Work out the finished part from the listing and answer in its coordinate system (mm). A direction names the side the tool comes from. Round coordinates to 2 decimals unless told otherwise and drop trailing zeros. Write each loop counter-clockwise with the first axis right and the second up, starting at its lowest first coordinate (ties: lowest second). Pieces come first, ordered by that corner, then holes.
from build123d import *

# Parameters (mm, degrees)
SKETCH_1_W                                = 111
SKETCH_1_H                                = 84
BOTTOM_LOWER_BASE_PLATE_3MM_DEPTH         = 3
SKETCH_3_R                                = 3
BOTTOM_LOWER_SCREW_6MM_THROUGH_DEPTH      = 3
SKETCH_5_R                                = 16.5
BOTTOM_LOWER_BATTERY_CLEARANCE_33MM_DEPTH = 3
SKETCH_7_W                                = 23
SKETCH_7_H                                = 23
BOTTOM_LOWER_BUZZER_POCKET_1P5MM_DEPTH    = 1.5
BOTTOM_LOWER_BUZZER_SOUND_HOLES_3MM_START = 1.5
SKETCH_9_R                                = 1.5
BOTTOM_LOWER_BUZZER_SOUND_HOLES_3MM_DEPTH = 1.5


with BuildPart() as part:
    # Эскиз1 → bottom_lower_base_plate_3mm (new body)
    with BuildSketch(Plane.XY):
        with Locations((53.5, 40)):
            Rectangle(SKETCH_1_W, SKETCH_1_H)
    extrude(amount=BOTTOM_LOWER_BASE_PLATE_3MM_DEPTH)

    # Эскиз3 → bottom_lower_screw_6mm_through (cut)
    with BuildSketch(Plane.XY):
        with Locations(Location((11.04, 7.54, 0), (0, 0, 180))):
            Circle(SKETCH_3_R)
        with Locations(Location((95.96, 7.54, 0), (0, 0, 180))):
            Circle(SKETCH_3_R)
        with Locations(Location((11.04, 72.46, 0), (0, 0, 180))):
            Circle(SKETCH_3_R)
        with Locations(Location((95.96, 72.46, 0), (0, 0, 180))):
            Circle(SKETCH_3_R)
    extrude(amount=BOTTOM_LOWER_SCREW_6MM_THROUGH_DEPTH, mode=Mode.SUBTRACT)

    # Эскиз5 → bottom_lower_battery_clearance_33mm (cut)
    with BuildSketch(Plane.XY):
        with Locations(Location((58.8, 24.5, 0), (0, 0, 180))):
            Circle(SKETCH_5_R)
    extrude(amount=BOTTOM_LOWER_BATTERY_CLEARANCE_33MM_DEPTH, mode=Mode.SUBTRACT)

    # Эскиз7 → bottom_lower_buzzer_pocket_1p5mm (cut)
    with BuildSketch(Plane.XY):
        with Locations((32.4, 17.3)):
            Rectangle(SKETCH_7_W, SKETCH_7_H)
    extrude(amount=BOTTOM_LOWER_BUZZER_POCKET_1P5MM_DEPTH, mode=Mode.SUBTRACT)

    # Эскиз9 → bottom_lower_buzzer_sound_holes_3mm (cut)
    with BuildSketch(Plane.XY.offset(BOTTOM_LOWER_BUZZER_SOUND_HOLES_3MM_START)):
        with Locations(Location((27.4, 12.3, 0), (0, 0, 180))):
            Circle(SKETCH_9_R)
        with Locations(Location((27.4, 17.3, 0), (0, 0, 180))):
            Circle(SKETCH_9_R)
        with Locations(Location((27.4, 22.3, 0), (0, 0, 180))):
            Circle(SKETCH_9_R)
        with Locations(Location((32.4, 12.3, 0), (0, 0, 180))):
            Circle(SKETCH_9_R)
        with Locations(Location((32.4, 17.3, 0), (0, 0, 180))):
            Circle(SKETCH_9_R)
        with Locations(Location((32.4, 22.3, 0), (0, 0, 180))):
            Circle(SKETCH_9_R)
        with Locations(Location((37.4, 12.3, 0), (0, 0, 180))):
            Circle(SKETCH_9_R)
        with Locations(Location((37.4, 17.3, 0), (0, 0, 180))):
            Circle(SKETCH_9_R)
        with Locations(Location((37.4, 22.3, 0), (0, 0, 180))):
            Circle(SKETCH_9_R)
    extrude(amount=BOTTOM_LOWER_BUZZER_SOUND_HOLES_3MM_DEPTH, mode=Mode.SUBTRACT)


solid = part.part
Q1. Find section D-D (x = 27.4). Determine the outline of the cut face in (y, z), plus the area to 3 significant figures.
Q2. The mould has two halves that part along Y. Classify faces 3 (the face through (53, 41, 0)), 4 (the face through (53, 82, 1)), 5 (the face through (33.51, 21.29, 2.24)): +Y half, -Y half, draft (parallel to the pull), parting line (faces both ways), or undercut.
Q3. A tool of negligible diameter and unlimited length cuts with its end or side. For faces 1 (the face through (38.51, 16.29, 2.24)), 2 (the face through (30, 17, 1.5)), from which of +Z, -Z, +X, -X, +Y, -Y can it reach the whole face along a straight path? Write none if from no direction.
Q4. Find section C-C (x = 95.96). Determine the outline of the cut face in (y, z).
Q5. Given pin 1 (5 mm diameter, centred on x = 27.4, y = 12.3, fed in from -Z), flat-ended and moving along its own axis, determine where the tip first touches the part or whether it passes through.
Q6. Find section B-B (z = 0.85). Determine the outline of the cut face in (x, y), plus the area to 3 significant figures.
Q7. Find the intervals of material crossed by L1, parallel to Y at x = 37.4, z = 2.15; L2, parallel to X at y = 17.3, z = 2.1; L3, parallel to X at y = 12, z = 2.25, in increasing order.
Q8. Find section A-A (x = 58.8). Determine the outline of the cut face in (y, z).
Report:
1. outline: (-2, 0) - (5.8, 0) - (5.8, 1.5) - (10.8, 1.5) - (10.8, 3) - (-2, 3) - close; (13.8, 1.5) - (15.8, 1.5) - (15.8, 3) - (13.8, 3) - close; (18.8, 1.5) - (20.8, 1.5) - (20.8, 3) - (18.8, 3) - close; (23.8, 1.5) - (28.8, 1.5) - (28.8, 0) - (82, 0) - (82, 3) - (23.8, 3) - close
1. area: 204 mm2
2. face 3: draft
2. face 4: +Y half
2. face 5: undercut
3. face 1: +Z, -Z
3. face 2: -Z
4. outline: (-2, 0) - (4.54, 0) - (4.54, 3) - (-2, 3) - close; (10.54, 0) - (69.46, 0) - (69.46, 3) - (10.54, 3) - close; (75.46, 0) - (82, 0) - (82, 3) - (75.46, 3) - close
5. pin 1: stops at z = 1.5
6. outline: (-2, -2) - (109, -2) - (109, 82) - (-2, 82) - close; hole circle Ø6 at (11.04, 7.54); hole circle Ø6 at (11.04, 72.46); hole (20.9, 5.8) - (43.9, 5.8) - (43.9, 17.41) arc R16.5 ccw (long way) to (42.87, 28.8) - (20.9, 28.8) - close; hole circle Ø6 at (95.96, 7.54); hole circle Ø6 at (95.96, 72.46)
6. area: 7,840 mm2
7. L1: y = -2 to 10.8, 13.8 to 15.8, 18.8 to 20.8, 23.8 to 82
7. L2: x = -2 to 25.9, 28.9 to 30.9, 33.9 to 35.9, 38.9 to 43.95, 73.65 to 109
7. L3: x = -2 to 25.93, 28.87 to 30.93, 33.87 to 35.93, 38.87 to 48.03, 69.57 to 109
8. outline: (-2, 0) - (8, 0) - (8, 3) - (-2, 3) - close; (41, 0) - (82, 0) - (82, 3) - (41, 3) - close
